Here's how the part is built. I have some questions about the finished solid (model axes, mm). Face numbers are marked on the shaded views. A direction names the side the tool comes from. Round coordinates to 2 decimals unless told otherwise and drop trailing zeros. Order: outer loops, then holes, each group sorted by start corner. A loop starts at its lowest first (then second) coordinate and runs counter-clockwise, first axis right, second up. Notation, with made-up numbers: (63, 42) - (121, 42) arc R29 ccw to (121, 66) - close; hole circle Ø10 at (-32, 78). An arc over 180 degrees is marked (long way). Answer as a JSON object with one key per item and string values.
```python
from build123d import *

# Parameters (mm, degrees)
F0_R     = 22.45
F1_DEPTH = 5
F2_W     = 32
F2_H     = 21.45
F2_H_2   = 32
F2_W_2   = 21.45
F3_DEPTH = 2.5
F4_R     = 1.6
F4_R_2   = 0.75
F5_DEPTH = 4


with BuildPart() as f1:
    # F0 (on Top) → F1 (new body)
    with BuildSketch(Plane.XY):
        Circle(F0_R)
    extrude(amount=F1_DEPTH)

    # F2 (on Top) → F3 (join)
    with BuildSketch(Plane.XY):
        with Locations((0, 26.725)):
            Rectangle(F2_W, F2_H)
        Rectangle(F2_W, F2_H_2)
        with Locations((-26.725, 0)):
            Rectangle(F2_W_2, F2_H_2)
        with Locations((26.725, 0)):
            Rectangle(F2_W_2, F2_H_2)
        with Locations((0, -26.725)):
            Rectangle(F2_W, F2_H)
    extrude(amount=-F3_DEPTH)

    # F4 (on face) → F5 (join)
    with BuildSketch(Plane.XY.offset(5)):
        with Locations((12.5612070115, 12.3107198171)):
            Circle(F4_R)
        with Locations((12.5612070115, 12.3107198171)):
            Circle(F4_R_2, mode=Mode.SUBTRACT)
        with Locations((-12.5387929885, 12.3107198171)):
            Circle(F4_R)
        with Locations((-12.5387929885, 12.3107198171)):
            Circle(F4_R_2, mode=Mode.SUBTRACT)
        with Locations((-12.5387929885, -12.2892801829)):
            Circle(F4_R)
        with Locations((-12.5387929885, -12.2892801829)):
            Circle(F4_R_2, mode=Mode.SUBTRACT)
        with Locations((12.5612070115, -12.2892801829)):
            Circle(F4_R)
        with Locations((12.5612070115, -12.2892801829)):
            Circle(F4_R_2, mode=Mode.SUBTRACT)
    extrude(amount=F5_DEPTH)


solid = f1.part
```
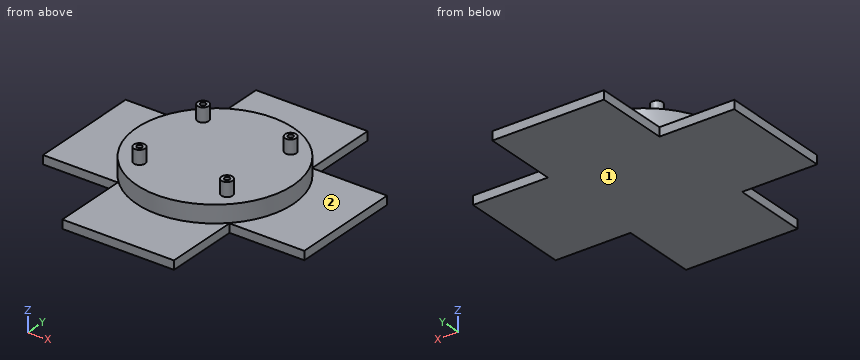
1. For the marked faces 1 and 2, which set-ups out of +Z, -Z, +X, -X, +Y, -Y let a thin tool reach every point of the face, with its end or its side?
Responses:
{"face 1": "-Z, +X, -X, +Y, -Y", "face 2": "+Z"}
2. Imagine slicing it at B-B (x = 0). List the corners of the cut face in (y, z) for me.
Responses:
{"outline": "(-37.45, -2.5) - (37.45, -2.5) - (37.45, 0) - (22.45, 0) - (22.45, 5) - (-22.45, 5) - (-22.45, 0) - (-37.45, 0) - close"}
3. Imagine slicing it at A-A (z = -1.25). List the corners of the cut face in (x, y) for me.
Responses:
{"outline": "(-37.45, -16) - (-16, -16) - (-16, -37.45) - (16, -37.45) - (16, -16) - (37.45, -16) - (37.45, 16) - (16, 16) - (16, 37.45) - (-16, 37.45) - (-16, 16) - (-37.45, 16) - close"}
4. If I drill on L1, parallel to Z at x = 1.5, y = 8; L2, parallel to Z at x = 30.5, y = 4.5; L3, parallel to Y at x = 22, z = -0.5, over which ranges is the centre line in solid material (lowest first)? Write a range as [from, to].
Responses:
{"L1": "[-2.5, 5]", "L2": "[-2.5, 0]", "L3": "[-16, 16]"}
5. Imagine slicing it at D-D (y = 26). List the corners of the cut face in (x, z) for me, plus the area to 3 significant figures.
Responses:
{"outline": "(-16, -2.5) - (16, -2.5) - (16, 0) - (-16, 0) - close", "area": "80.0 mm2"}
6. For P1, Ø1, axis at x = 24, y = 1, coming from the +Z side; P2, Ø12, axis at x = 12, y = 24.5, coming from the +Z side; P3, Ø0.8, axis at y = 29, z = -1.5, coming from the -X side, each with a flat end and sliding along its axis, tell me the tip position at first contact or that it passes through.
Responses:
{"P1": "z = 0", "P2": "z = 5", "P3": "x = -16"}
